Autodesk Inventor part; units mm, degrees
ref_plane "Plano de trabajo1" through (0, 2.375, 0) normal (0, 1, 0) x (1, 0, 0)
ref_plane "YZ Plane" through (0, 0, 0) normal (1, 0, 0) x (0, 1, 0)
ref_plane "XZ Plane" through (0, 0, 0) normal (0, 1, 0) x (-1, 0, 0)
sketch "Boceto1" plane through (0, 0, 0) normal (0, 1, 0) x (-1, 0, 0)
  line L0 (-2.125, 2.625) -> (2.125, 2.625)
  line L1 (2.625, 2.125) -> (2.625, -2.125)
  line L2 (2.125, -2.625) -> (-2.125, -2.625)
  line L3 (-2.625, -2.125) -> (-2.625, 2.125)
  line L4 (-2.625, 2.625) -> (2.625, -2.625) construction
  line L5 (2.625, 2.625) -> (-2.625, -2.625) construction
  arc A0 (2.625, 2.125) -> (2.125, 2.625) centre (2.125, 2.125) ccw
  arc A1 (2.125, -2.625) -> (2.625, -2.125) centre (2.125, -2.125) ccw
  arc A2 (-2.625, -2.125) -> (-2.125, -2.625) centre (-2.125, -2.125) ccw
  arc A3 (-2.125, 2.625) -> (-2.625, 2.125) centre (-2.125, 2.125) ccw
  point P0 (0, 0)
  point P1 (0, -2.625)
  dimension "d0" = 0.5
  dimension "d1" = 5.25
  dimension "d2" = 5.25
extrude "Extrusión1" add sketch "Boceto1" along normal blind 0.5
sketch "Boceto2" plane through (0, 0.5, 0) normal (0, 1, 0) x (1, 0, 0)
  line L0 (1.875, -1.875) -> (-1.875, -1.875)
  line L1 (-1.875, -1.875) -> (-1.875, 1.875)
  line L2 (-1.875, 1.875) -> (1.875, 1.875)
  line L3 (1.875, 1.875) -> (1.875, -1.875)
  line L4 (1.875, -1.875) -> (-1.875, 1.875) construction
  line L5 (-1.875, -1.875) -> (1.875, 1.875) construction
  point P0 (0, 0)
  dimension "d5" = 3.75
  dimension "d6" = 3.75
ref_plane "Plano de trabajo1" through (0, 2.375, 0) normal (0, 1, 0) x (1, 0, 0)
sketch "Boceto3" plane through (0, 2.375, 0) normal (0, 1, 0) x (1, 0, 0)
  line L0 (0.9375, -0.9375) -> (-0.9375, -0.9375)
  line L1 (-0.9375, -0.9375) -> (-0.9375, 0.9375)
  line L2 (-0.9375, 0.9375) -> (0.9375, 0.9375)
  line L3 (0.9375, 0.9375) -> (0.9375, -0.9375)
  line L4 (0.9375, -0.9375) -> (-0.9375, 0.9375) construction
  line L5 (-0.9375, -0.9375) -> (0.9375, 0.9375) construction
  point P0 (0, 0)
  dimension "d8" = 1.875
  dimension "d9" = 1.875
loft "Solevación1" add profiles "Boceto2", "Boceto3"
sketch "Boceto4" plane through (-0.9375, 2.375, 0.9375) normal (0, 1, 0) x (1, 0, 0)
  line L0 (1.875, 0) -> (0, 0)
  line L1 (1.875, 1.875) -> (1.875, 0)
  line L2 (0, 1.875) -> (1.875, 1.875)
  line L3 (0, 0) -> (0, 1.875)
  point P0 (0.9375, 0.9375)
extrude "Extrusión2" add sketch "Boceto4" along normal blind 0.75
shell "Vaciado5" thickness 0.375 removed faces 1 at (0.3125, 3.125, 0.3125)
sketch "Boceto11" plane through (0, 0, 0) normal (0, 0, 1) x (1, 0, 0)
  line L0 (1.5182, 0.375) -> (0.5625, 2.2865)
  line L1 (-1.5182, 0.375) -> (-0.5625, 2.2865)
  line L2 (1.5182, 0.375) -> (1.7057, 0)
  line L3 (-1.5182, 0.375) -> (-1.7057, 0)
  line L4 (1.7057, 0) -> (-1.7057, 0)
  point P0 (0, 0)
  point P1 (-2.625, 0)
sketch "Boceto10" plane through (0, 0, 0) normal (0, -1, 0) x (1, 0, 0)
  line L0 (1.7057, 1.7057) -> (-1.7057, 1.7057)
  line L1 (-1.7057, 1.7057) -> (-1.7057, -1.7057)
  line L2 (-1.7057, -1.7057) -> (1.7057, -1.7057)
  line L3 (1.7057, -1.7057) -> (1.7057, 1.7057)
  line L4 (1.7057, 1.7057) -> (-1.7057, -1.7057) construction
  line L5 (-1.7057, 1.7057) -> (1.7057, -1.7057) construction
  point P0 (0, 0)
  point P1 (-1.7057, 0)
  point P2 (-1.7057, 0)
sketch "Boceto12" plane through (-1.5182, 0.375, -1.5182) normal (0, 1, 0) x (1, 0, 0)
  line L0 (3.0365, -3.0365) -> (3.0365, 0)
  line L1 (3.0365, 0) -> (0, 0)
  line L2 (0, 0) -> (0, -3.0365)
  line L3 (0, -3.0365) -> (3.0365, -3.0365)
  point P0 (1.5182, -1.5182)
loft "Solevación3" cut profiles "Boceto10" section 1 edges at (1.5182, 0.375, 0) (0, 0.375, -1.5182) (-1.5182, 0.375, 0) (0, 0.375, 1.5182)
equation "\"d6\" = d5"
equation "\"d9\" = d8"
properties part number "ejercicio_clase_5"
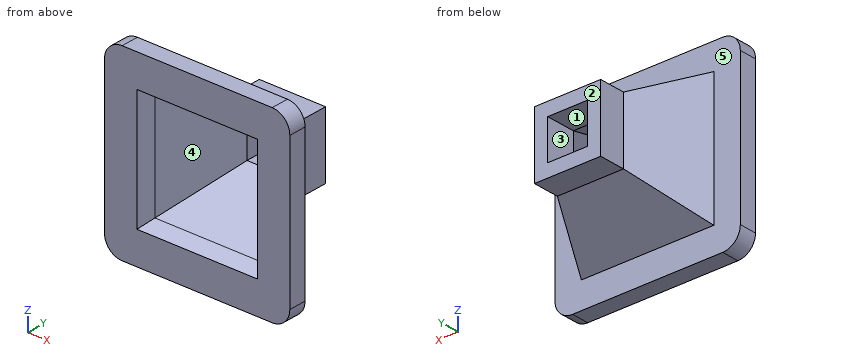
Here's how the part is built. I have some questions about the finished solid (model axes, mm). Face numbers are marked on the shaded views. A direction names the side the tool comes from. Round coordinates to 2 decimals unless told otherwise and drop trailing zeros. Order: outer loops, then holes, each group sorted by start corner. A loop starts at its lowest first (then second) coordinate and runs counter-clockwise, first axis right, second up. Notation, with made-up numbers: M 30.25,47 L 71.25,47 A25 cw 71.25,86 Z; hole C 13,77 d8. An arc over 180 degrees is marked long. Answer in a Markdown table with one row per item.
Item 1: Thinking about a two-plate mould opening in X: for the marked faces 1 and 2, which applies, +X half, -X half, draft (parallel to the pull), parting line (faces both ways), or undercut?
A:
| item | result |
|---|---|
| face 1 | undercut |
| face 2 | draft |
Item 2: I'm going to push flat-ended pins straight in: pin 1 (0.8 mm diameter, centred on x = -0.5, y = 3, fed in from -Z); pin 2 (1.5 mm diameter, centred on x = -1, y = 2, fed in from -Z); pin 3 (0.7 mm diameter, centred on y = 3, z = 0, fed in from -X). Where does each tip first touch, or does it pass through?
A:
| item | result |
|---|---|
| pin 1 | stops at z = -0.94 |
| pin 2 | stops at z = -1.5 |
| pin 3 | stops at x = -0.94 |
Item 3: If I drill on L1, parallel to Z at x = 0.5, y = 2.95; L2, parallel to Z at x = -0.2, y = 0.9 (3 decimals), over which ranges is the centre line in solid material (lowest first)? Write a range as from..to.
A:
| item | result |
|---|---|
| L1 | z = -0.94..-0.56, 0.56..0.94 |
| L2 | z = -1.675..-1.256, 1.256..1.675 |
Item 4: For the marked faces 3, 4 and 5, which set-ups out of +Z, -Z, +X, -X, +Y, -Y let a thin tool reach every point of the face, with its end or its side?
A:
| item | result |
|---|---|
| face 3 | +Y, -Y |
| face 4 | -Y |
| face 5 | +Y |
Item 5: Imagine slicing it at A-A, the plane y = 2.85. Write out the boundary of the cut face in (x, z).
A:
| item | result |
|---|---|
| outline | M -0.94,-0.94 L 0.94,-0.94 L 0.94,0.94 L -0.94,0.94 Z; hole M -0.56,-0.56 L 0.56,-0.56 L 0.56,0.56 L -0.56,0.56 Z |
Item 6: Imagine slicing it at B-B, the plane z = 1.95. Write out the boundary of the cut face in (x, y) (3 decimals), and give its area (4 significant figures).
A:
| item | result |
|---|---|
| outline | M -2.625,0 L 2.625,0 L 2.625,0.5 L -2.625,0.5 Z |
| area | 2.625 mm2 |
